For this review, take the finished solid that the model builds, in its own axes (mm). A direction names the side the tool comes from. Round coordinates to 2 decimals unless told otherwise and drop trailing zeros. Answer in a Markdown table with one row per item.
from build123d import *

# Parameters (mm, degrees)
F0_R     = 11.075
F1_DEPTH = 7
F2_R     = 2
F4_DEPTH = 25


# Not quite as in the source:
# - a feature names something its author has since deleted; it is built from what else it names


with BuildPart() as f1:
    # F0 (on Top) → F1 (new body)
    with BuildSketch(Plane.XY):
        with BuildLine():
            ThreePointArc((10.8590541373, 28.4748429105), (9.3936805028, 22.9693269387), (5.3853374572, 18.9207207546))
            Line((5.3853374572, 18.9207207546), (6.5097166395, 17.0028645343))
            Line((6.5097166395, 17.0028645343), (13.0819100939, 20.7973221943))
            Line((13.0819100939, 20.7973221943), (13.0819100939, 36.1523636266))
            Line((13.0819100939, 36.1523636266), (-0.2159458627, 43.8298843428))
            Line((-0.2159458627, 43.8298843428), (-13.5138018192, 36.1523636266))
            Line((-13.5138018192, 36.1523636266), (-13.5138018192, 20.7973221943))
            Line((-13.5138018192, 20.7973221943), (-6.7881393171, 16.9142591382))
            Line((-6.7881393171, 16.9142591382), (-5.6894167006, 18.8469281837))
            ThreePointArc((-5.6894167006, 18.8469281837), (-5.7853684301, 38.0475727858), (10.8590541373, 28.4748429105))
        make_face()
        with BuildLine():
            Line((6.5097166395, 17.0028645343), (5.3853374572, 18.9207207546))
            ThreePointArc((5.3853374572, 18.9207207546), (-0.1421532918, 17.4000887526), (-5.6894167006, 18.8469281837))
            Line((-5.6894167006, 18.8469281837), (-6.7881393171, 16.9142591382))
            Line((-6.7881393171, 16.9142591382), (-0.2159458627, 13.1198014782))
            Line((-0.2159458627, 13.1198014782), (6.5097166395, 17.0028645343))
        make_face()
        Polygon((18.1892172392, -2.9188871567), (6.5097166395, 17.0028645343), (-0.2159458627, 13.1198014782), (-6.7881393171, 16.9142591382), (-18.2011320695, -3.1613609301), (-11.4686565798, -7.0562964045), (-11.4753544728, -14.6335356233), (11.6169113166, -14.4796687622), (11.5092421808, -6.9031915863), align=None)
        with Locations((-0.0247963396, -0.2127871583)):
            Circle(F0_R, mode=Mode.SUBTRACT)
        with BuildLine():
            Line((19.313711516, -4.836939694), (18.1892172392, -2.9188871567))
            Line((18.1892172392, -2.9188871567), (11.5092421808, -6.9031915863))
            Line((11.5092421808, -6.9031915863), (11.6169113166, -14.4796687622))
            Line((11.6169113166, -14.4796687622), (13.840240678, -14.4648544208))
            ThreePointArc((13.840240678, -14.4648544208), (15.2870801091, -8.917591012), (19.313711516, -4.836939694))
        make_face()
        with BuildLine():
            Line((-11.4686565798, -7.0562964045), (-18.2011320695, -3.1613609301))
            Line((-18.2011320695, -3.1613609301), (-19.2999671542, -5.0942278088))
            ThreePointArc((-19.2999671542, -5.0942278088), (-15.2193158362, -9.1208592157), (-13.6986838342, -14.6483499647))
            Line((-13.6986838342, -14.6483499647), (-11.4753544728, -14.6335356233))
            Line((-11.4753544728, -14.6335356233), (-11.4686565798, -7.0562964045))
        make_face()
        with BuildLine():
            Line((-19.2999671542, -5.0942278088), (-18.2011320695, -3.1613609301))
            Line((-18.2011320695, -3.1613609301), (-24.759864777, 0.6330592247))
            Line((-24.759864777, 0.6330592247), (-38.0646461892, -7.0327869064))
            Line((-38.0646461892, -7.0327869064), (-38.0782194043, -22.3879886667))
            Line((-38.0782194043, -22.3879886667), (-24.7870112072, -30.077344296))
            Line((-24.7870112072, -30.077344296), (-11.4822297949, -22.4114981649))
            Line((-11.4822297949, -22.4114981649), (-11.4753544728, -14.6335356233))
            Line((-11.4753544728, -14.6335356233), (-13.6986838342, -14.6483499647))
            ThreePointArc((-13.6986838342, -14.6483499647), (-13.6984994528, -14.6852460454), (-13.6984379921, -14.7221425356))
            ThreePointArc((-13.6984379921, -14.7221425356), (-34.3461678674, -20.2915651031), (-19.2999671542, -5.0942278088))
        make_face()
        with BuildLine():
            Line((24.6968043769, 0.9625956381), (18.1892172392, -2.9188871567))
            Line((18.1892172392, -2.9188871567), (19.313711516, -4.836939694))
            ThreePointArc((19.313711516, -4.836939694), (30.4205108077, -4.7814354844), (35.9899948359, -14.3910618499))
            ThreePointArc((35.9899948359, -14.3910618499), (24.9518913261, -25.4660003892), (13.840240678, -14.4648544208))
            Line((13.840240678, -14.4648544208), (11.6169113166, -14.4796687622))
            Line((11.6169113166, -14.4796687622), (11.7274326398, -22.2568490742))
            Line((11.7274326398, -22.2568490742), (25.1331852948, -29.7447193378))
            Line((25.1331852948, -29.7447193378), (38.3207474909, -21.8789321135))
            Line((38.3207474909, -21.8789321135), (38.1025570319, -6.5252746256))
            Line((38.1025570319, -6.5252746256), (24.6968043769, 0.9625956381))
        make_face()
    extrude(amount=F1_DEPTH)

    # F2
    f2_edges = [f1.edges().sort_by_distance(p)[0] for p in [
        (-10.150971, 18.855791, 7),
        (-13.513802, 28.474843, 7),
        (-6.864874, 39.991124, 7),
        (6.432982, 39.991124, 7),
        (13.08191, 28.474843, 7),
        (12.349467, 7.041989, 7),
        (9.795813, 18.900093, 7),
        (21.443011, -0.978146, 7),
        (31.399681, -2.781339, 7),
        (38.211652, -14.202103, 7),
        (31.726966, -25.811826, 7),
        (18.430309, -26.000784, 7),
        (11.672172, -18.368259, 7),
        (0.070778, -14.556602, 7),
        (-11.478792, -18.522517, 7),
        (-31.432615, -26.232666, 7),
        (-18.134621, -26.244421, 7),
        (-38.071433, -14.710388, 7),
        (-31.412255, -3.199864, 7),
        (-21.480498, -1.264151, 7),
        (-12.494636, 6.876449, 7),
        (31.726966, -25.811826, 0),
        (38.211652, -14.202103, 0),
        (31.399681, -2.781339, 0),
        (21.443011, -0.978146, 0),
        (18.430309, -26.000784, 0),
        (11.672172, -18.368259, 0),
        (12.349467, 7.041989, 0),
        (0.070778, -14.556602, 0),
        (9.795813, 18.900093, 0),
        (13.08191, 28.474843, 0),
        (6.432982, 39.991124, 0),
        (-6.864874, 39.991124, 0),
        (-13.513802, 28.474843, 0),
        (-10.150971, 18.855791, 0),
        (-12.494636, 6.876449, 0),
        (-21.480498, -1.264151, 0),
        (-31.412255, -3.199864, 0),
        (-38.071433, -14.710388, 0),
        (-31.432615, -26.232666, 0),
        (-18.134621, -26.244421, 0),
        (-11.478792, -18.522517, 0),
    ]]
    fillet(f2_edges, radius=F2_R)

    # F3 (on face) → F4 (cut)
    with BuildSketch(Plane.XY.offset(7)):
        Polygon((1.443375673, 16.7368283158), (-1.443375673, 16.7368283158), (-2.8867513459, 14.2368283158), (-1.443375673, 11.7368283158), (1.443375673, 11.7368283158), (2.8867513459, 14.2368283158), align=None)
        Polygon((-10.8739663642, -5.3167335935), (-13.7607177101, -5.3167335935), (-15.2040933831, -7.8167335935), (-13.7607177101, -10.3167335935), (-10.8739663642, -10.3167335935), (-9.4305906912, -7.8167335935), align=None)
        Polygon((13.7978978307, -5.1664386955), (10.9111464847, -5.1664386955), (9.4677708117, -7.6664386955), (10.9111464847, -10.1664386955), (13.7978978307, -10.1664386955), (15.2412735036, -7.6664386955), align=None)
    extrude(amount=-F4_DEPTH, mode=Mode.SUBTRACT)


solid = f1.part
1) Consider section A-A on x = 8.5. State how many separate pieces and enclosed holes the cut face has, then the cut area to 3 significant figures.
Solved:
| item | result |
|---|---|
| separate pieces | 4 |
| enclosed holes | 0 |
| area | 138 mm² |
2) Mouldability with a two-part tool opening along Y and no side actions: class faces 4 (the cylindrical face through (-12.94, 28.37, 0.6)), 5 (the cylindrical face through (6.05, 39.55, 6.4)), 6 (the cylindrical face through (31.527, -25.267, 0.601)), 7 (the cylindrical face through (11.76, 6.92, 0.6)) as pulls with the +Y half, pulls with the -Y half, needs draft (parallel to the pull), parting line crosses it, or undercut.
Solved:
| item | result |
|---|---|
| face 4 | needs draft |
| face 5 | pulls with the +Y half |
| face 6 | pulls with the -Y half |
| face 7 | undercut |
3) For line 1 (Y direction, x = -6, z = 2); line 2 (X direction, y = -1, z = 1); line 3 (Y direction, x = -0.5, z = 1.5), list the stretches that pass through material, from the lowest coordinate up. Write a range as [from, to].
Solved:
| item | result |
|---|---|
| line 1 | [-14.6, -9.54], [9.11, 19.03], [37.92, 40.49] |
| line 2 | [-27.06, -22.47], [-16.66, -11.07], [11.02, 16.75], [21.93, 27.66] |
| line 3 | [-14.5, -11.28], [10.85, 11.74], [16.74, 17.4], [39.55, 43.59] |
4) For faces 1 (the flat face through (21.49, -0.95, 3.48)), 2 (the cylindrical face through (12.51, 28.58, 0.6)), 3 (the cylindrical face through (-21, -2.2, 6.4)), list the 3-axis set-ups (+Z, -Z, +X, -X, +Y, -Y) from which the entire face can be reached by the end or side of a thin tool; tool diameter is ignored.
Solved:
| item | result |
|---|---|
| face 1 | +Z, -Z, +Y |
| face 2 | -Z, +X, +Y |
| face 3 | +Z, +Y |
5) Clearance check with flat-ended pins moving along their axes: pin 1 Ø2.5 at (x, z) = (-0.5, 3) entering from +Y; pin 2 Ø1 at (x, z) = (-19.5, 5.5) entering from -Y; pin 3 Ø2.5 at (y, z) = (30.5, 3) entering from -X; pin 4 Ø2.5 at (x, z) = (12, 2) entering from +Y. State where each tip first meets the part, or that it passes through.
Solved:
| item | result |
|---|---|
| pin 1 | y = 43.83 |
| pin 2 | y = -27.27 |
| pin 3 | x = -13.51 |
| pin 4 | y = 37.5 |
